from build123d import *

# Parameters (mm, degrees)
SKETCH1_W           = 88.9
SKETCH1_H           = 76.2
SKETCH1_W_2         = 53.65
SKETCH1_H_2         = 15.65
BOSS_EXTRUDE1_DEPTH = 3.175
SKETCH2_W           = 5.334
SKETCH2_H           = 3.302
SKETCH2_W_2         = 3.302
SKETCH2_H_2         = 5.334
CUT_EXTRUDE1_DEPTH  = 59.630138368


with BuildPart() as part:
    # Sketch1 → Boss-Extrude1 (new body)
    with BuildSketch(Plane(origin=(0, 0, 0), x_dir=(1, 0, 0), z_dir=(0, 1, 0))):
        Rectangle(SKETCH1_W, SKETCH1_H)
        with Locations((-7.465, 0)):
            Rectangle(SKETCH1_W_2, SKETCH1_H_2, mode=Mode.SUBTRACT)
    extrude(amount=BOSS_EXTRUDE1_DEPTH)

    # Sketch2 → Cut-Extrude1 (cut, through all)
    with BuildSketch(Plane(origin=(0, 0, 0), x_dir=(1, 0, 0), z_dir=(0, 1, 0))):
        with Locations((-25.4, -36.449)):
            Rectangle(SKETCH2_W, SKETCH2_H)
        with Locations((-42.799, -15.24)):
            Rectangle(SKETCH2_W_2, SKETCH2_H_2)
        with Locations((-42.799, -25.4)):
            Rectangle(SKETCH2_W_2, SKETCH2_H_2)
        with Locations((-42.799, -5.08)):
            Rectangle(SKETCH2_W_2, SKETCH2_H_2)
        with Locations((-42.799, 5.08)):
            Rectangle(SKETCH2_W_2, SKETCH2_H_2)
        with Locations((-42.799, 15.24)):
            Rectangle(SKETCH2_W_2, SKETCH2_H_2)
        with Locations((-42.799, 25.4)):
            Rectangle(SKETCH2_W_2, SKETCH2_H_2)
        with Locations((42.799, 25.4)):
            Rectangle(SKETCH2_W_2, SKETCH2_H_2)
        with Locations((42.799, 15.24)):
            Rectangle(SKETCH2_W_2, SKETCH2_H_2)
        with Locations((42.799, 5.08)):
            Rectangle(SKETCH2_W_2, SKETCH2_H_2)
        with Locations((42.799, -5.08)):
            Rectangle(SKETCH2_W_2, SKETCH2_H_2)
        with Locations((42.799, -15.24)):
            Rectangle(SKETCH2_W_2, SKETCH2_H_2)
        with Locations((42.799, -25.4)):
            Rectangle(SKETCH2_W_2, SKETCH2_H_2)
        with Locations((-15.24, -36.449)):
            Rectangle(SKETCH2_W, SKETCH2_H)
        with Locations((-5.08, -36.449)):
            Rectangle(SKETCH2_W, SKETCH2_H)
        with Locations((5.08, -36.449)):
            Rectangle(SKETCH2_W, SKETCH2_H)
        with Locations((15.24, -36.449)):
            Rectangle(SKETCH2_W, SKETCH2_H)
        with Locations((25.4, -36.449)):
            Rectangle(SKETCH2_W, SKETCH2_H)
        with Locations((25.4, 36.449)):
            Rectangle(SKETCH2_W, SKETCH2_H)
        with Locations((15.24, 36.449)):
            Rectangle(SKETCH2_W, SKETCH2_H)
        with Locations((5.08, 36.449)):
            Rectangle(SKETCH2_W, SKETCH2_H)
        with Locations((-5.08, 36.449)):
            Rectangle(SKETCH2_W, SKETCH2_H)
        with Locations((-15.24, 36.449)):
            Rectangle(SKETCH2_W, SKETCH2_H)
        with Locations((-25.4, 36.449)):
            Rectangle(SKETCH2_W, SKETCH2_H)
    extrude(amount=CUT_EXTRUDE1_DEPTH, mode=Mode.SUBTRACT)


solid = part.part
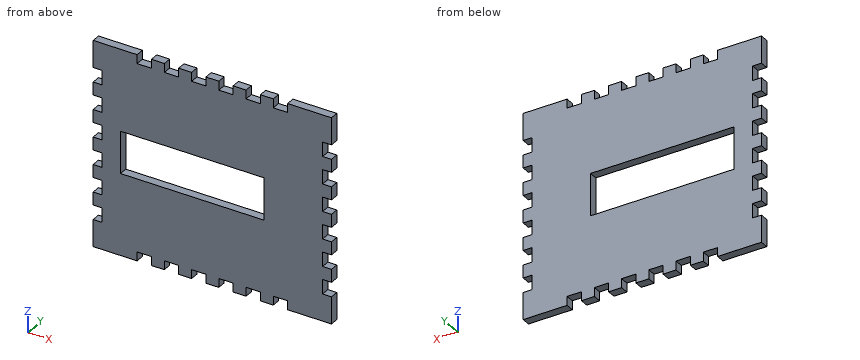
For this review, take the finished solid that the model builds, in its own axes (mm). Coordinates: 2 decimals unless noted, no trailing zeros. Loops run counter-clockwise (first coordinate to the right, second up) from the corner with the lowest first, then second, coordinate; pieces in that order, holes last. Notation, with made-up numbers: (80, 59) - (101, 59) arc R28 ccw to (101, 94) - close; hole circle Ø6 at (2.25, -24.75). An arc over 180 degrees is marked (long way). Use a Markdown table: item, result. Add a question column.
Item 1: We need section C-C (z = -26). Give the boundary of the cut face in (x, y) (3 decimals), and give its area (3 significant figures).
Item 2: We need section B-B (x = 24). Give the boundary of the cut face in (y, z) (3 decimals).
Item 3: For line 1 (Z direction, x = -4, y = 2.8) (3 decimals); line 2 (X direction, y = 1.8, z = 0); line 3 (X direction, y = 0.5, z = 4), list the stretches that pass through material, from the lowest coordinate up.
Item 4: Insertion check: pin 1 Ø1.6 at (y, z) = (2.5, -4) entering from +X; pin 2 Ø1.6 at (x, y) = (24.5, 1) entering from -Z; pin 3 Ø1 at (x, y) = (-4.5, 1) entering from +Z. Each pin has a flat end and moves straight along its axis. Give the tip position at first contact, or say it passes through.
Item 5: We need section A-A (x = -24.5). Give the boundary of the cut face in (y, z) (3 decimals).
Results list:
| question | item | result |
|---|---|---|
| 1 | outline | (-41.148, 0) - (41.148, 0) - (41.148, 3.175) - (-41.148, 3.175) - close |
| 1 | area | 261 mm^2 |
| 2 | outline | (0, -34.798) - (3.175, -34.798) - (3.175, 34.798) - (0, 34.798) - close |
| 3 | line 1 | z = -34.798 to -7.825, 7.825 to 34.798 |
| 3 | line 2 | x = -44.45 to -34.29, 19.36 to 44.45 |
| 3 | line 3 | x = -41.15 to -34.29, 19.36 to 41.15 |
| 4 | pin 1 | stops at x = 41.15 |
| 4 | pin 2 | stops at z = -34.8 |
| 4 | pin 3 | stops at z = 34.8 |
| 5 | outline | (0, -34.798) - (3.175, -34.798) - (3.175, -7.825) - (0, -7.825) - close; (0, 7.825) - (3.175, 7.825) - (3.175, 34.798) - (0, 34.798) - close |
